Autodesk Inventor part; units mm, degrees
ref_plane "РабПлоскость1" through (-126, 0, 110) normal (0, 0, 1) x (1, 0, 0)
ref_plane "РабПлоскость2" through (-96, 0, 220) normal (1, 0, 0) x (0, 0, -1)
ref_plane "YZ Plane" through (0, 0, 0) normal (1, 0, 0) x (0, 1, 0)
sketch "Эскиз1" plane through (0, 0, 0) normal (0, 1, 0) x (-1, 0, 0)
  line L0 (0, 220) -> (192, 220)
  line L1 (192, 220) -> (192, 0)
  line L2 (192, 0) -> (0, 0)
  line L3 (0, 0) -> (0, 220)
  circle A0 centre (11, 217) radius 1.5
  circle A1 centre (181, 217) radius 1.5
  circle A2 centre (5, 3) radius 1.5
  circle A3 centre (187, 3) radius 1.5
  line L4 (186, 6) -> (6, 6)
  line L5 (6, 6) -> (6, 244)
  line L6 (6, 244) -> (186, 244)
  line L7 (186, 244) -> (186, 6)
  dimension "d0" = 192
  dimension "d1" = 170
  dimension "d2" = 220
  dimension "d3" = 11
  dimension "d4" = 3
  dimension "d5" = 3
  dimension "d6" = 3
  dimension "d7" = 3
  dimension "d8" = 3
  dimension "d9" = 5
  dimension "d10" = 3
  dimension "d11" = 3
  dimension "d12" = 5
  dimension "d13" = 3
  dimension "d16" = 238
  dimension "d18" = 180
  dimension "d19" = 6
  dimension "d20" = 6
extrude "Выдавливание2" add sketch "Эскиз1" along normal blind 6 contours L0 L5 L4 L7 L1 L2 L3 | L0 L7 L4 L5 | A0 | A1 | A2 | A3
sketch "Эскиз2" plane through (0, 0, 0) normal (0, -1, 0) x (1, 0, 0)
  line L0 (-192, 220) -> (0, 220)
  line L1 (-6, 220) -> (-26, 220)
  line L2 (-26, 220) -> (-26, 214)
  line L3 (-26, 214) -> (-6, 214)
  line L4 (-6, 214) -> (-6, 220)
  line L5 (-46, 220) -> (-66, 220)
  line L6 (-66, 220) -> (-66, 214)
  line L7 (-66, 214) -> (-46, 214)
  line L8 (-46, 214) -> (-46, 220)
  line L9 (-186, 220) -> (-166, 220)
  line L10 (-166, 220) -> (-166, 214)
  line L11 (-166, 214) -> (-186, 214)
  line L12 (-186, 214) -> (-186, 220)
  line L13 (-146, 220) -> (-126, 220)
  line L14 (-126, 220) -> (-126, 214)
  line L15 (-126, 214) -> (-146, 214)
  line L16 (-146, 214) -> (-146, 220)
  line L17 (0, 220) -> (0, 0)
  line L18 (-192, 0) -> (-192, 220)
  point P0 (-66, 217)
  point P1 (-46, 217)
  point P2 (-26, 217)
  point P3 (-146, 217)
  point P4 (-126, 217)
  point P5 (-166, 217)
  point P6 (-186, 217)
  point P7 (-166, 220)
  point P8 (-126, 220)
  dimension "d23" = 6
  dimension "d24" = 20
  dimension "d25" = 6
  dimension "d26" = 20
  dimension "d27" = 20
  dimension "d28" = 20
  dimension "d29" = 20
  dimension "d30" = 20
  dimension "d31" = 6
extrude "Выдавливание3" cut sketch "Эскиз2" against normal through all
ref_plane "РабПлоскость1" through (-126, 0, 110) normal (0, 0, 1) x (1, 0, 0)
mirror "Зеркальное отражение1" about plane through (-126, 0, 110) normal (0, 0, 1) of "Выдавливание3"
sketch "Эскиз3" plane through (0, 0, 0) normal (0, -1, 0) x (1, 0, 0)
  circle A0 centre (-3, 98.5) radius 1.5
  circle A1 centre (-3, 121.5) radius 1.5
  circle A2 centre (-189, 98.5) radius 1.5
  circle A3 centre (-189, 121.5) radius 1.5
  line L0 (-192, 0) -> (-192, 220)
  line L1 (-231.3831, 110) -> (44.2986, 110)
  line L2 (0, 220) -> (0, 0)
  dimension "d34" = 3
  dimension "d35" = 3
  dimension "d36" = 3
  dimension "d37" = 11.5
  dimension "d38" = 3
  dimension "d39" = 11.5
  dimension "d40" = 3
  dimension "d41" = 3
  dimension "d43" = 11.5
  dimension "d44" = 3
  dimension "d45" = 3
  dimension "d46" = 11.5
extrude "Выдавливание4" cut sketch "Эскиз3" against normal blind 10
sketch "Эскиз4" plane through (0, 6, 0) normal (0, 1, 0) x (1, 0, 0)
  line L0 (4.3155, -27.8106) -> (4.3155, -29.0145)
  line L1 (4.3155, -43.2101) -> (4.3155, -29.2101)
  line L2 (4.3155, -31.8771) -> (4.3155, -40.1101)
  line L3 (4.3155, -27.8106) -> (4.3155, -29.0145)
  circle A0 centre (-3, -121.5) radius 1.5
  circle A1 centre (-189, -121.5) radius 1.5
  circle A2 centre (-3, -98.5) radius 1.5
  circle A3 centre (-189, -98.5) radius 1.5
  line L4 (-126, 0) -> (-126, -6)
  line L5 (-126, -6) -> (-146, -6)
  line L6 (-146, -6) -> (-146, 0)
  line L7 (-146, 0) -> (-166, 0)
  line L8 (-166, 0) -> (-166, -6)
  line L9 (-166, -6) -> (-186, -6)
  line L10 (-186, -6) -> (-186, 0)
  line L11 (-186, 0) -> (-192, 0)
  line L12 (-192, 0) -> (-192, -220)
  line L13 (-192, -220) -> (-186, -220)
  line L14 (-186, -220) -> (-186, -214)
  line L15 (-186, -214) -> (-166, -214)
  line L16 (-166, -214) -> (-166, -220)
  line L17 (-166, -220) -> (-146, -220)
  line L18 (-146, -220) -> (-146, -214)
  line L19 (-146, -214) -> (-126, -214)
  line L20 (-126, -214) -> (-126, -220)
  line L21 (-126, -220) -> (-66, -220)
  line L22 (-66, -220) -> (-66, -214)
  line L23 (-66, -214) -> (-46, -214)
  line L24 (-46, -214) -> (-46, -220)
  line L25 (-46, -220) -> (-26, -220)
  line L26 (-26, -220) -> (-26, -214)
  line L27 (-26, -214) -> (-6, -214)
  line L28 (-6, -214) -> (-6, -220)
  line L29 (-6, -220) -> (0, -220)
  line L30 (0, -220) -> (0, 0)
  line L31 (0, 0) -> (-6, 0)
  line L32 (-6, 0) -> (-6, -6)
  line L33 (-6, -6) -> (-26, -6)
  line L34 (-26, -6) -> (-26, 0)
  line L35 (-26, 0) -> (-46, 0)
  line L36 (-46, 0) -> (-46, -6)
  line L37 (-46, -6) -> (-66, -6)
  line L38 (-66, -6) -> (-66, 0)
  line L39 (-66, 0) -> (-126, 0)
  line L40 (0, -27.5) -> (0, -30.5)
  line L41 (-6, -30.5) -> (-6, -27.5)
  line L42 (0, -27.5) -> (0, -30.5)
  line L43 (-6, -30.5) -> (-6, -27.5)
  line L44 (0, -41.5) -> (0, -44.5)
  line L45 (-6, -44.5) -> (-6, -41.5)
  line L46 (0, -29) -> (0, -43)
  line L47 (-6, -43) -> (-6, -29)
  line L48 (0, -41.5) -> (0, -44.5)
  line L49 (-6, -44.5) -> (-6, -41.5)
  line L50 (4.3155, -22.5218) -> (4.3155, -51.048)
  line L51 (4.9155, -36.9084) -> (0.7155, -36.9084)
  line L52 (4.3155, -22.5218) -> (4.3155, -51.048)
  line L53 (1.3155, -44.914) -> (1.3155, -41.914)
  line L54 (4.3155, -44.914) -> (4.3155, -41.914)
  line L55 (4.3155, -43.6493) -> (1.3155, -43.6493)
  line L56 (4.3155, -40.543) -> (1.3155, -40.543)
  line L57 (1.3155, -40.543) -> (1.3155, -46.3135)
  line L58 (4.3155, -40.543) -> (4.3155, -46.3135)
  line L59 (1.3155, -32.3101) -> (1.3155, -40.543)
  line L60 (4.3155, -43.4057) -> (4.3155, -44.6096)
  line L61 (4.3155, -32.3101) -> (1.3155, -32.3101)
  line L62 (4.3155, -32.3101) -> (4.3155, -40.543)
  line L63 (1.3155, -30.9201) -> (1.3155, -27.9201)
  line L64 (4.3155, -30.9201) -> (4.3155, -27.9201)
  line L65 (1.3155, -26.5206) -> (1.3155, -32.3101)
  line L66 (4.3155, -26.5206) -> (4.3155, -32.3101)
  line L67 (4.3155, -31.8771) -> (1.3155, -31.8771)
  line L68 (4.3155, -28.7709) -> (1.3155, -28.7709)
  line L69 (1.3155, -31.8771) -> (1.3155, -40.1101)
  line L70 (4.3155, -31.8771) -> (4.3155, -40.1101)
  line L71 (1.3155, -43.2101) -> (1.3155, -29.2101)
  line L72 (4.3155, -43.2101) -> (4.3155, -29.2101)
  line L73 (1.3155, -26.1066) -> (1.3155, -31.8771)
  line L74 (4.3155, -26.1066) -> (4.3155, -31.8771)
  line L75 (1.3155, -43.4057) -> (1.3155, -44.6096)
  line L76 (1.3155, -44.5) -> (1.3155, -41.5)
  line L77 (4.3155, -44.5) -> (4.3155, -41.5)
  line L78 (4.3155, -43.4057) -> (1.3155, -43.4057)
  line L79 (4.3155, -40.1101) -> (1.3155, -40.1101)
  line L80 (1.3155, -40.1101) -> (1.3155, -45.8995)
  line L81 (4.3155, -40.1101) -> (4.3155, -45.8995)
  line L82 (1.3155, -30.5061) -> (1.3155, -27.5061)
  line L83 (4.3155, -29.0145) -> (1.3155, -29.0145)
  line L84 (4.3155, -27.8106) -> (4.3155, -29.0145)
  line L85 (4.3155, -30.5061) -> (4.3155, -27.5061)
  line L86 (1.3155, -27.8106) -> (1.3155, -29.0145)
  line L87 (4.3155, -41.914) -> (4.3155, -44.914)
  line L88 (4.3155, -40.5145) -> (4.3155, -46.3135)
  line L89 (4.3155, -43.3697) -> (4.3155, -43.0444)
  line L90 (4.3155, -41.5) -> (4.3155, -44.5)
  line L91 (4.3155, -40.1005) -> (4.3155, -45.8995)
  line L92 (4.3155, -22.2315) -> (4.3155, -52.6365) construction
  line L93 (4.3155, -23.5797) -> (4.3155, -51.7445) construction
  line L94 (4.3155, -35.5823) -> (4.3155, -36.4187)
  line L95 (4.3155, -30.9195) -> (4.3155, -41.9147)
  line L96 (4.3155, -42.8814) -> (4.3155, -43.61) construction
  line L97 (4.3155, -29.0505) -> (4.3155, -29.2131)
  line L98 (4.3155, -29.2101) -> (4.3155, -43.2101)
  line L99 (4.3155, -27.8106) -> (4.3155, -44.6096)
  line L100 (4.3155, -28.8799) -> (4.3155, -29.6854) construction
  line L101 (4.3155, -29.3758) -> (4.3155, -29.2131)
  line L102 (4.3155, -27.9201) -> (4.3155, -30.9201)
  line L103 (4.3155, -26.5206) -> (4.3155, -32.3196)
  line L104 (4.3155, -27.5061) -> (4.3155, -30.5061)
  line L105 (4.3155, -26.1066) -> (4.3155, -31.9056)
  line L106 (4.3155, -30.5055) -> (4.3155, -36.0031)
  line L107 (4.3155, -41.5007) -> (4.3155, -36.0031)
  line L108 (4.3155, -29.6845) -> (4.3155, -30.2653) construction
  point P0 (4.3155, -43.414)
  point P1 (4.3155, -43)
  point P2 (4.3155, -36.2101)
  point P3 (4.3155, -29.4201)
  point P4 (4.3155, -29.0061)
  point P5 (4.3155, -35.9427)
  point P6 (4.3155, -31.8212)
sketch "Эскиз5" plane through (0, 6, 0) normal (0, 1, 0) x (1, 0, 0)
  circle A0 centre (-172, -41) radius 1.5
  circle A1 centre (-172, -31) radius 1.5
  line L0 (-186, -214) -> (-166, -214)
  line L1 (-192, 0) -> (-192, -220)
  line L2 (-166, -6) -> (-186, -6)
  circle A2 centre (-147, -41) radius 1.5
  circle A3 centre (-147, -31) radius 1.5
  point P0 (0, 0)
  dimension "d49" = 3
  dimension "d52" = 20
  dimension "d53" = 10
  dimension "d54" = 3
  dimension "d57" = 25
  dimension "d58" = 20
  dimension "d87" = 3
  dimension "d88" = 25
  dimension "d89" = 25
extrude "Выдавливание5" cut sketch "Эскиз5" against normal blind 10
ref_plane "РабПлоскость2" through (-96, 0, 220) normal (1, 0, 0) x (0, 0, -1)
mirror "Зеркальное отражение2" about plane through (-96, 0, 220) normal (1, 0, 0) of "Выдавливание5"
sketch "Эскиз6" plane through (-126, 0, 220) normal (0, 0, 1) x (1, 0, 0)
  line L0 (-66, 6) -> (126, 6)
  line L1 (126, 6) -> (126, 0)
  line L2 (126, 0) -> (-66, 0)
  line L3 (-66, 0) -> (-66, 6)
  line L4 (-66, 6) -> (-60, 6)
  line L5 (-60, 6) -> (-60, 0)
  line L6 (-60, 0) -> (-66, 0)
  line L7 (-66, 0) -> (-66, 6)
  line L8 (-40, 6) -> (-20, 6)
  line L9 (-20, 6) -> (-20, 0)
  line L10 (-20, 0) -> (-40, 0)
  line L11 (-40, 0) -> (-40, 6)
  line L12 (0, 6) -> (60, 6)
  line L13 (60, 6) -> (60, 0)
  line L14 (60, 0) -> (0, 0)
  line L15 (0, 0) -> (0, 6)
  line L16 (80, 6) -> (100, 6)
  line L17 (100, 6) -> (100, 0)
  line L18 (100, 0) -> (80, 0)
  line L19 (80, 0) -> (80, 6)
  line L20 (120, 6) -> (126, 6)
  line L21 (126, 6) -> (126, 0)
  line L22 (126, 0) -> (120, 0)
  line L23 (120, 0) -> (120, 6)
  line L24 (-66, 6) -> (-60, 6)
  line L25 (-60, 6) -> (-60, 0)
  line L26 (-60, 0) -> (-66, 0)
  line L27 (-40, 6) -> (-20, 6)
  line L28 (-20, 6) -> (-20, 0)
  line L29 (-20, 0) -> (-40, 0)
  line L30 (-40, 0) -> (-40, 6)
  line L31 (0, 6) -> (60, 6)
  line L32 (60, 6) -> (60, 0)
  line L33 (60, 0) -> (0, 0)
  line L34 (0, 0) -> (0, 6)
  line L35 (80, 6) -> (100, 6)
  line L36 (100, 6) -> (100, 0)
  line L37 (100, 0) -> (80, 0)
  line L38 (80, 0) -> (80, 6)
  line L39 (120, 6) -> (126, 6)
  line L40 (126, 6) -> (126, 0)
  line L41 (126, 0) -> (120, 0)
  line L42 (120, 0) -> (120, 6)
  line L43 (-66, 6) -> (-60, 6)
  line L44 (-60, 6) -> (-60, 0)
  line L45 (-60, 0) -> (-66, 0)
  line L46 (-40, 6) -> (-20, 6)
  line L47 (-20, 6) -> (-20, 0)
  line L48 (-20, 0) -> (-40, 0)
  line L49 (-40, 0) -> (-40, 6)
  line L50 (0, 6) -> (60, 6)
  line L51 (60, 6) -> (60, 0)
  line L52 (60, 0) -> (0, 0)
  line L53 (0, 0) -> (0, 6)
  line L54 (80, 6) -> (100, 6)
  line L55 (100, 6) -> (100, 0)
  line L56 (100, 0) -> (80, 0)
  line L57 (80, 0) -> (80, 6)
  line L58 (120, 6) -> (126, 6)
  line L59 (126, 6) -> (126, 0)
  line L60 (126, 0) -> (120, 0)
  line L61 (120, 0) -> (120, 6)
  line L62 (120, 6) -> (126, 6)
  line L63 (126, 0) -> (126, 6)
  line L64 (120, 0) -> (126, 0)
  line L65 (-66, 0) -> (-66, 6)
  line L66 (-66, 0) -> (-66, 6)
extrude "Выдавливание6" add sketch "Эскиз6" along normal blind 6
sketch "Эскиз7" plane through (0, 0, 0) normal (0, -1, 0) x (1, 0, 0)
  circle A0 centre (-3, 12.5) radius 1.5
  line L0 (0, 0) -> (0, 226)
  line L1 (-26, 6) -> (-6, 6)
  circle A1 centre (-189, 12.5) radius 1.5
  line L2 (-192, 0) -> (-192, 226)
  line L3 (-186, 6) -> (-166, 6)
  dimension "d61" = 3
  dimension "d62" = 3
  dimension "d64" = 6.5
  dimension "d65" = 3
  dimension "d66" = 3
  dimension "d67" = 6.5
extrude "Выдавливание7" cut sketch "Эскиз7" against normal through all
sketch "Эскиз8" plane through (0, 0, 0) normal (0, -1, 0) x (1, 0, 0)
  circle A0 centre (-11, 167) radius 1.5
  circle A1 centre (-11, 72) radius 1.5
  circle A2 centre (-156, 167) radius 1.5
  circle A3 centre (-156, 72) radius 1.5
  line L0 (-46, 220) -> (-26, 220)
  line L1 (-166, 214) -> (-186, 214)
  line L2 (0, 0) -> (0, 226)
  dimension "d70" = 95
  dimension "d71" = 95
  dimension "d72" = 145
  dimension "d73" = 3
  dimension "d74" = 3
  dimension "d75" = 3
  dimension "d76" = 3
  dimension "d77" = 53
  dimension "d78" = 47
  dimension "d79" = 11
  dimension "d80" = 11
  dimension "d81" = 145
extrude "Выдавливание8" cut sketch "Эскиз8" against normal through all
equation "\"d39\" = d37"
equation "\"d43\" = d37"
equation "\"d46\" = d37"
equation "\"d74\" = d73"
equation "\"d75\" = d73"
equation "\"d76\" = d73"
properties part number "дно_пробитое"
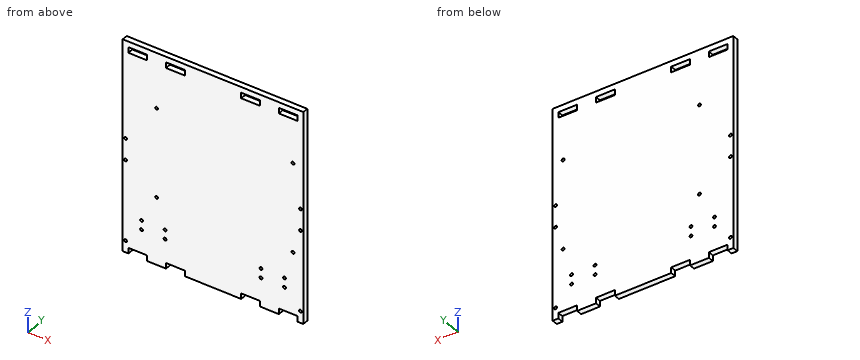
The listing builds one solid part. Answer for the finished solid, in the listing's coordinates (mm). Give positions to 0.01 mm unless a question says otherwise; leave off trailing zeros. Order: outer loops, then holes, each group sorted by start corner. A loop starts at its lowest first (then second) coordinate and runs counter-clockwise, first axis right, second up.
Item 1: The part is cut by section A-A, the plane x = -50.5. Give the vertices of the cut face in (y, z), and give its area (3 significant figures).
From the geometry:
outline: (0, 6) - (6, 6) - (6, 214) - (0, 214) - close; (0, 220) - (6, 220) - (6, 226) - (0, 226) - close
area: 1,280 mm2
Item 2: Find the intervals of material crossed by probe 1 along Z at (x, y) = (-147, 4.05); probe 2 along X at (y, z) = (3.45, 98.5); probe 3 along X at (y, z) = (3, 72), in increasing order.
From the geometry:
probe 1: z = 0 to 29.5, 32.5 to 39.5, 42.5 to 226
probe 2: x = -192 to -190.5, -187.5 to -4.5, -1.5 to 0
probe 3: x = -192 to -157.5, -154.5 to -12.5, -9.5 to 0
Item 3: The part is cut by section B-B, the plane y = 4. Count the separate pieces of the cut face and the enclosed holes in it, and give its area (3 significant figures).
From the geometry:
separate pieces: 1
enclosed holes: 22
area: 42,300 mm2
Item 4: Given pin 1 Ø1.8 at (x, y) = (-14, 2.5) entering from -Z, flat-ended and moving along its own axis, determine where the tip first touches the part or whether it passes through.
From the geometry:
pin 1: stops at z = 6
